```python
from build123d import *

# Parameters (mm, degrees)
F0_W      = 140
F0_H      = 80
F1_DEPTH  = 35
F2_W      = 100
F2_H      = 9
F3_DEPTH  = 10
F5_R      = 5
F6_R      = 5
F7_R      = 7.5
F8_DEPTH  = 1
F9_W      = 5
F9_H      = 5
F10_DEPTH = 1


with BuildPart() as f1:
    # F0 (on Top) → F1 (new body)
    with BuildSketch(Plane.XY):
        with Locations((5.1616433263, -11.4978505671)):
            Rectangle(F0_W, F0_H)
    extrude(amount=F1_DEPTH)

    # F2 (on face) → F3 (cut)
    with BuildSketch(Plane.XZ.offset(51.4978505671)):
        with Locations((5.1616433263, 14.5)):
            Rectangle(F2_W, F2_H)
    extrude(amount=-F3_DEPTH, mode=Mode.SUBTRACT)

    # F5
    f5_edges = [f1.edges().sort_by_distance(p)[0] for p in [
        (75.161643, -11.497851, 0),
        (5.161643, -51.497851, 0),
        (5.161643, 28.502149, 0),
        (-64.838357, -11.497851, 0),
    ]]
    fillet(f5_edges, radius=F5_R)

    # F6
    f6_edges = [f1.edges().sort_by_distance(p)[0] for p in [
        (-64.838357, -11.497851, 35),
        (5.161643, 28.502149, 35),
        (5.161643, -51.497851, 35),
        (75.161643, -11.497851, 35),
    ]]
    fillet(f6_edges, radius=F6_R)

    # F7 (on face) → F8 (join)
    with BuildSketch(Plane.XZ.offset(51.4978505671)):
        with Locations((-56.063328834, 15.5)):
            Circle(F7_R)
    extrude(amount=F8_DEPTH)

    # F9 (on face) → F10 (cut)
    with BuildSketch(Plane.XZ.offset(52.4978505671)):
        with Locations((-55.7435365021, 14.7882593423)):
            Rectangle(F9_W, F9_H)
    extrude(amount=-F10_DEPTH, mode=Mode.SUBTRACT)


solid = f1.part
```
Work out the finished part from the listing and answer in its coordinate system (mm). A direction names the side the tool comes from. Give positions to 0.01 mm unless a question says otherwise; leave off trailing zeros. Loops run counter-clockwise (first coordinate to the right, second up) from the corner with the lowest first, then second, coordinate; pieces in that order, holes last. Notation, with made-up numbers: (3.25, -28.75) -> (47.25, -28.75) arc R8 cw to (47.25, -19.75) -> close; hole circle Ø2 at (58.5, 27). An arc over 180 degrees is marked (long way). One line per question, with ' | ' between items. Start each with the question number.
1) Section A-A, the plane x = 65 is taken. Determine the outline of the cut face in (y, z), then the cut area to 3 significant figures.
2) For faces 5 (the face through (-48.91, -51.99, 17.75)), 6 (the face through (73.66, -10.94, 1.43)), determine the directions among +Z, -Z, +X, -X, +Y, -Y from which every point of the face is accessible in a straight line to the end or side of a thin tool.
3) Section B-B, the plane z = 15.5 is taken. Determine the outline of the cut face in (x, y).
4) Each of these flat-tipped pins is pushed along its axis until it touches: pin 1 (4.5 mm diameter, centred on x = -0.5, z = 16, fed in from -Y); pin 2 (2.5 mm diameter, centred on x = -56, z = 15, fed in from -Y); pin 3 (0.5 mm diameter, centred on x = -55, y = -52, fed in from -Z). Where does it stop, or does it pass through?
5) Section C-C, the plane x = -6.5 is taken. Determine the outline of the cut face in (y, z), then the cut area to 3 significant figures.
6) Determine the mould class of faces 1 (the face through (6.142, 26.999, 33.574)), 2 (the face through (73.66, -10.94, 33.57)), 3 (the face through (4, -47, 19)), 4 (the face through (4, -47, 10)) for opening direction X: +X half, -X half, draft (parallel to the pull), parting line (faces both ways), or undercut.
7) Straight lines are drawn through the part: L1, parallel to Z at x = 5, y = -42.5; L2, parallel to Y at x = -21, z = 9.5; L3, parallel to Y at x = 32, z = 17. For each, find the intervals that lie inside material, in ascending order.
Resolved:
1) outline: (-51.5, 5) arc R5 ccw to (-46.5, 0) -> (23.5, 0) arc R5 ccw to (28.5, 5) -> (28.5, 30) arc R5 ccw to (23.5, 35) -> (-46.5, 35) arc R5 ccw to (-51.5, 30) -> close | area: 2,780 mm2
2) face 5: -Y | face 6: -Z, +X, +Y, -Y
3) outline: (-64.84, -51.5) -> (-63.56, -51.5) -> (-63.56, -52.5) -> (-58.24, -52.5) -> (-58.24, -51.5) -> (-53.24, -51.5) -> (-53.24, -52.5) -> (-48.56, -52.5) -> (-48.56, -51.5) -> (-44.84, -51.5) -> (-44.84, -41.5) -> (55.16, -41.5) -> (55.16, -51.5) -> (75.16, -51.5) -> (75.16, 28.5) -> (-64.84, 28.5) -> close
4) pin 1: y = -41.5 | pin 2: y = -51.5 | pin 3: z = 8.04
5) outline: (-51.5, 5) arc R5 ccw to (-46.5, 0) -> (23.5, 0) arc R5 ccw to (28.5, 5) -> (28.5, 30) arc R5 ccw to (23.5, 35) -> (-46.5, 35) arc R5 ccw to (-51.5, 30) -> (-51.5, 19) -> (-41.5, 19) -> (-41.5, 10) -> (-51.5, 10) -> close | area: 2,690 mm2
6) face 1: draft | face 2: +X half | face 3: undercut | face 4: undercut
7) L1: 0 to 10, 19 to 35 | L2: -51.5 to 28.5 | L3: -41.5 to 28.5
